Job drawing, mm, ordinate dimensions from the low corner. One solid piece. A direction names the side the tool comes from. Round coordinates to 2 decimals unless told otherwise and drop trailing zeros. Loops run counter-clockwise (first coordinate to the right, second up) from the corner with the lowest first, then second, coordinate; pieces in that order, holes last. Notation, with made-up numbers: M 25,-17 L 61,-17 A18 cw 61,15 Z; hole C 45,-21.75 d1. An arc over 180 degrees is marked long. Use a Markdown table: item, result. Add a question column.
(1) Flat gauge pin, fed straight in: P1, Ø5, axis at x = 926.5, y = 602.5, coming from the -Z side. Where does the tip first touch, or does it go through?
(2) Two-plate mould, pull along Y, no slides. Class the marked faces 1, 2 and 3: released by +Y, released by -Y, zero draft, split by the parting line, or undercut.
(3) Band-saw the part on B-B, the plane x = 535. Write the cut outline in (y, z), and give its area (3 significant figures).
(4) Band-saw the part on A-A, the plane z = 136. Write the cut outline in (x, y).
(5) Band-saw the part on C-C, the plane y = 723.5. Write the cut outline in (x, z).
(6) Which spindle directions (+Z, -Z, +X, -X, +Y, -Y) get a long thin tool onto all of the face, cutting with end or side? Do the marked faces 4 and 5. Say none if no direction does.
(7) Wall check: L1, parallel to Y at x = 966.5, z = 35; L2, parallel to Z at x = 458, y = 697.5. Give the ranges that are in metal, low to high.
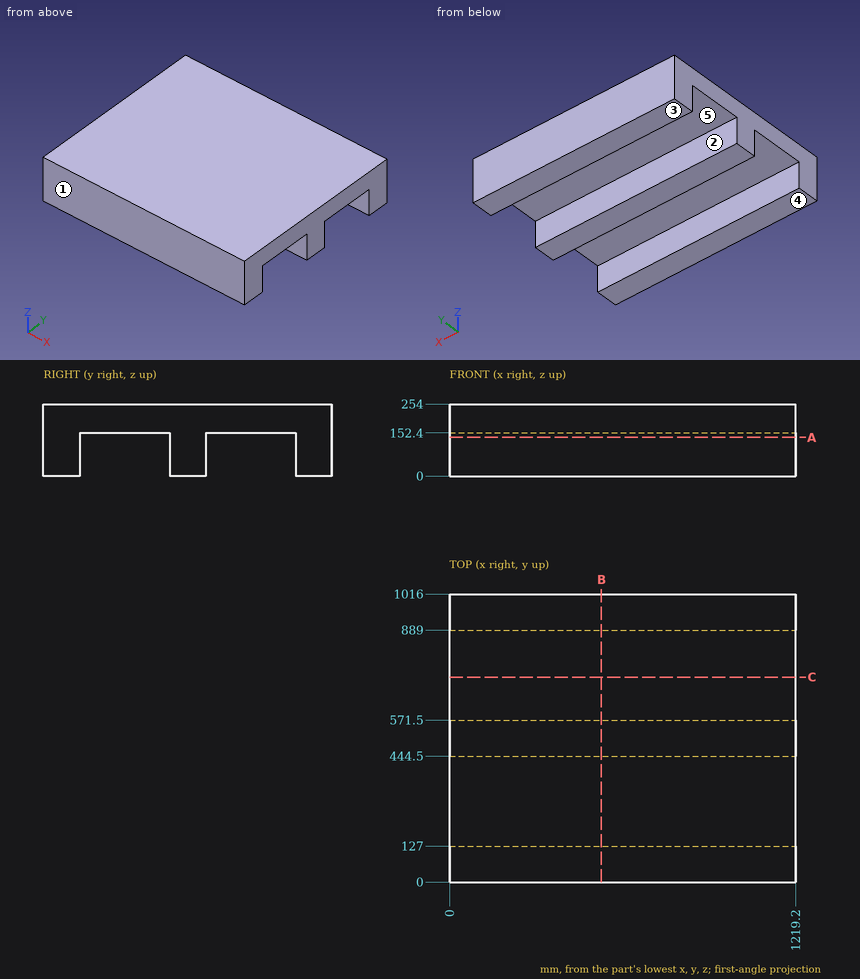
Return value:
| question | item | result |
|---|---|---|
| 1 | P1 | z = 152.4 |
| 2 | face 1 | released by -Y |
| 2 | face 2 | undercut |
| 2 | face 3 | zero draft |
| 3 | outline | M 0,0 L 127,0 L 127,152.4 L 444.5,152.4 L 444.5,0 L 571.5,0 L 571.5,152.4 L 889,152.4 L 889,0 L 1016,0 L 1016,254 L 0,254 Z |
| 3 | area | 161,000 mm^2 |
| 4 | outline | M 0,0 L 1219.2,0 L 1219.2,127 L 0,127 Z; M 0,444.5 L 1219.2,444.5 L 1219.2,571.5 L 0,571.5 Z; M 0,889 L 1219.2,889 L 1219.2,1016 L 0,1016 Z |
| 5 | outline | M 0,152.4 L 1219.2,152.4 L 1219.2,254 L 0,254 Z |
| 6 | face 4 | -Z, +X, -X, +Y, -Y |
| 6 | face 5 | -Z, +X, -X |
| 7 | L1 | 0 to 127, 444.5 to 571.5, 889 to 1016 |
| 7 | L2 | 152.4 to 254 |
